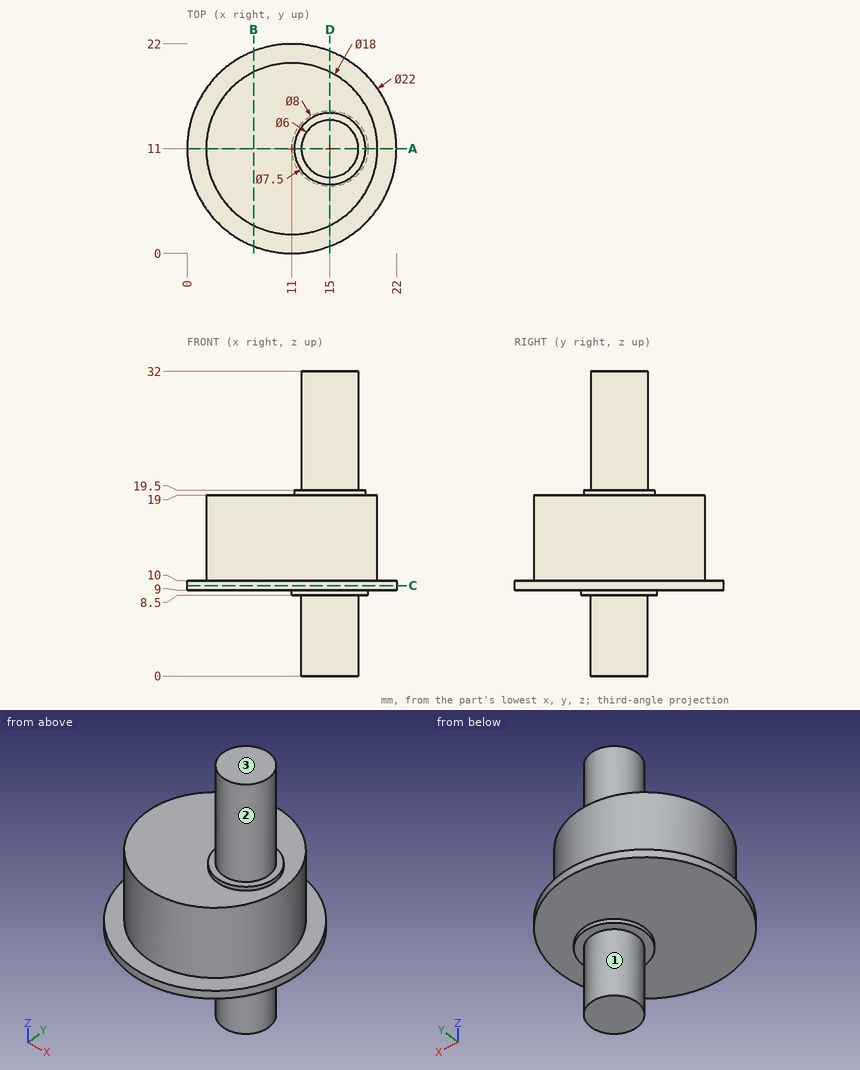
Source: three-view drawing plus pictorial views. Frame: mm from the lowest corner of the part. A direction names the side the tool comes from. Round coordinates to 2 decimals unless told otherwise and drop trailing zeros. Order: outer loops, then holes, each group sorted by start corner. A loop starts at its lowest first (then second) coordinate and runs counter-clockwise, first axis right, second up. Notation, with made-up numbers: (78, 85) - (107, 85) arc R26 cw to (107, 121) - close; hole circle Ø10 at (63.25, 77). An arc over 180 degrees is marked (long way). Use a Markdown table: item, result.
1. Section B-B on x = 7. Return the cut outline in (y, z).
Evaluation:
| item | result |
|---|---|
| outline | (0.75, 9) - (21.25, 9) - (21.25, 10) - (19.06, 10) - (19.06, 19) - (2.94, 19) - (2.94, 10) - (0.75, 10) - close |
2. First-contact query: pin 1 (11 mm diameter, centred on x = 8, y = 14, fed in from +Z); pin 2 (8 mm diameter, centred on y = 15.5, z = 20.5, fed in from +X); pin 3 (5 mm diameter, centred on x = 11, z = 6, fed in from -Y); pin 4 (12 mm diameter, centred on x = 9, y = 18, fed in from +Z). Flat tips, straight axial feed; report the tip coordinate or a pass-through.
Evaluation:
| item | result |
|---|---|
| pin 1 | z = 32 |
| pin 2 | x = 19.97 |
| pin 3 | y = 8.4 |
| pin 4 | z = 19.5 |
3. Section C-C on z = 9.5. Return the cut outline in (x, y), then the cut area to 3 significant figures.
Evaluation:
| item | result |
|---|---|
| outline | circle Ø22 at (11, 11) |
| area | 380 mm^2 |
4. Section D-D on x = 15. Return the cut outline in (y, z), then the cut area to 3 significant figures.
Evaluation:
| item | result |
|---|---|
| outline | (0.75, 9) - (7, 9) - (7, 8.5) - (8, 8.5) - (8, 0) - (14, 0) - (14, 8.5) - (15, 8.5) - (15, 9) - (21.25, 9) - (21.25, 10) - (19.06, 10) - (19.06, 19) - (14.75, 19) - (14.75, 19.5) - (14, 19.5) - (14, 32) - (8, 32) - (8, 19.5) - (7.25, 19.5) - (7.25, 19) - (2.94, 19) - (2.94, 10) - (0.75, 10) - close |
| area | 299 mm^2 |
5. Material intervals for probe 1 along Z at (x, y) = (6, 8.75); probe 2 along Z at (x, y) = (1.5, 11.5); probe 3 along Y at (x, z) = (9, 12), sorted ascending.
Evaluation:
| item | result |
|---|---|
| probe 1 | 9 to 19 |
| probe 2 | 9 to 10 |
| probe 3 | 2.23 to 19.77 |
6. Section A-A on y = 11. Return the cut outline in (x, z), then the cut area to 3 significant figures.
Evaluation:
| item | result |
|---|---|
| outline | (0, 9) - (11, 9) - (11, 8.5) - (12, 8.5) - (12, 0) - (18, 0) - (18, 8.5) - (19, 8.5) - (19, 9) - (22, 9) - (22, 10) - (20, 10) - (20, 19) - (18.75, 19) - (18.75, 19.5) - (18, 19.5) - (18, 32) - (12, 32) - (12, 19.5) - (11.25, 19.5) - (11.25, 19) - (2, 19) - (2, 10) - (0, 10) - close |
| area | 318 mm^2 |
7. Access query for the marked faces 1, 2 and 3. Directions: +Z, -Z, +X, -X, +Y, -Y. A direction counts if a zero-diameter tool reaches every point of the face in a straight line with its end or side. Return the directions, or none.
Evaluation:
| item | result |
|---|---|
| face 1 | -Z |
| face 2 | +Z |
| face 3 | +Z, +X, -X, +Y, -Y |
